```python
from build123d import *

# Parameters (mm, degrees)
F1_DEPTH = 25.4
F2_R     = 21.149451
F2_R_2   = 20.076598
F3_DEPTH = 25.4


with BuildPart() as f1:
    # F0 (on Top) → F1 (new body)
    with BuildSketch(Plane.XY):
        Polygon((-75.755887, 36.15994), (-75.755887, -75.42865), (77.392094, -75.42865), (68.556629, -29.287914), (-15.216626, -24.052085), (-28.306197, 19.797975), align=None)
    extrude(amount=F1_DEPTH)

    # F2 (on Top) → F3 (join)
    with BuildSketch(Plane.XY):
        with Locations((-49.765799, -71.501784)):
            Circle(F2_R)
        with Locations((43.749049, -71.333706)):
            Circle(F2_R_2)
    extrude(amount=F3_DEPTH)


solid = f1.part
```
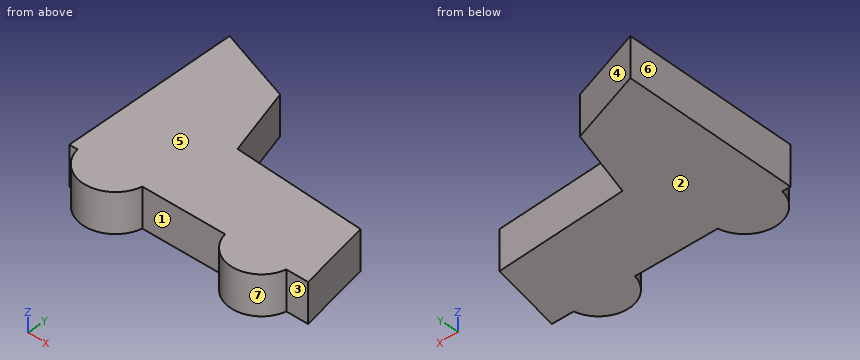
Part model, mm, in its own coordinate system. Face numbers are marked on the shaded views. A direction names the side the tool comes from. Round coordinates to 2 decimals unless told otherwise and drop trailing zeros. Order: outer loops, then holes, each group sorted by start corner. A loop starts at its lowest first (then second) coordinate and runs counter-clockwise, first axis right, second up. Notation, with made-up numbers: M -6,30.5 L 21,30.5 A33 ccw 21,58.5 Z; hole C 79,36.5 d1. An arc over 180 degrees is marked long. Answer in a Markdown table with one row per item. Add a question column.
Q1. Wall check: L1, parallel to Y at x = 68, z = 24.25; L2, parallel to X at y = -79.5, z = 21.5; L3, parallel to Y at x = 10, z = 19.5. Give the ranges that are in metal, low to high. Write a range as from..to.
Q2. Pin check, flat tips, straight feed: pin 1 (4 mm diameter, centred on x = 74, z = 10.5, fed in from -Y); pin 2 (5 mm diameter, centred on y = 9, z = 7.5, fed in from +X); pin 3 (5 mm diameter, centred on y = -12.5, z = 11.5, fed in from +X). Stop position of each tip, or through.
Q3. Cut at A-A on y = -84. Give the cut face in (x, z).
Q4. Cut at B-B on z = 18.5. Give the cut face in (x, y), and give its area (3 significant figures).
Q5. 3-axis set-ups, long thin cutter, end or side, ignore diameter. For the marked faces 1, 2 and 3: which of +Z, -Z, +X, -X, +Y, -Y reach the whole face in a straight line?
Q6. Cut at D-D on y = -50.5. Give the cut face in (x, z).
Q7. Mould opens along X. For the marked faces 4, 5, 6 and 7 say: +X half, -X half, draft (parallel to the pull), parting line (faces both ways), or undercut.
Q8. Cut at C-C on x = -33.5. Give the cut face in (y, z), and give its area (3 significant figures).
Established:
| question | item | result |
|---|---|---|
| 1 | L1 | y = -75.43..-29.25 |
| 1 | L2 | x = -69.34..-30.19, 25.41..62.09 |
| 1 | L3 | y = -75.43..-25.63 |
| 2 | pin 1 | stops at y = -75.43 |
| 2 | pin 2 | stops at x = -24.34 |
| 2 | pin 3 | stops at x = -17.92 |
| 3 | outline | M -66.83,0 L -32.7,0 L -32.7,25.4 L -66.83,25.4 Z; M 28.17,0 L 59.33,0 L 59.33,25.4 L 28.17,25.4 Z |
| 4 | outline | M -75.76,-75.43 L -70.55,-75.43 A21.15 ccw -28.98,-75.43 L 24.09,-75.43 A20.08 ccw 63.4,-75.43 L 77.39,-75.43 L 68.56,-29.29 L -15.22,-24.05 L -28.31,19.8 L -75.76,36.16 Z |
| 4 | area | 11,200 mm2 |
| 5 | face 1 | +Z, -Z, -Y |
| 5 | face 2 | -Z, +X, -X, +Y, -Y |
| 5 | face 3 | +Z, -Z, +X, -Y |
| 6 | outline | M -75.76,0 L 72.62,0 L 72.62,25.4 L -75.76,25.4 Z |
| 7 | face 4 | +X half |
| 7 | face 5 | draft |
| 7 | face 6 | -X half |
| 7 | face 7 | undercut |
| 8 | outline | M -85.02,0 L 21.59,0 L 21.59,25.4 L -85.02,25.4 Z |
| 8 | area | 2,710 mm2 |
